Geometry check sheet. Reference: the model listing, model coordinates, mm. Face numbers are marked on the shaded views. A direction names the side the tool comes from. Coordinates: 2 decimals unless noted, no trailing zeros. Order: outer loops, then holes, each group sorted by start corner. A loop starts at its lowest first (then second) coordinate and runs counter-clockwise, first axis right, second up. Notation, with made-up numbers: (0.25, -4.5) -> (16.25, -4.5) arc R28 ccw to (16.25, 19.5) -> close; hole circle Ø9 at (-19, -3.75). An arc over 180 degrees is marked (long way). Answer in a Markdown table with one row per item. Add a question column.
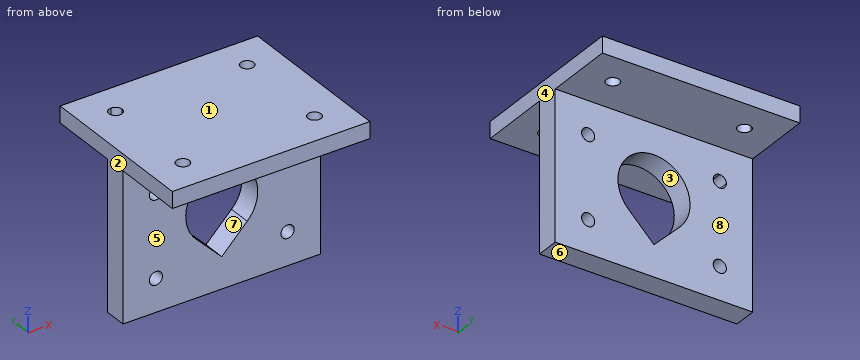
```python
from build123d import *

# Parameters (mm, degrees)
SKETCH_2_W           = 60
SKETCH_2_H           = 50
SKETCH_2_R           = 10.85
EXTRUDE_1_DEPTH      = 7
SKETCH_4_W           = 60
SKETCH_4_H           = 5
EXTRUDE_2_DEPTH      = 25
SKETCH_6_R           = 2
CUT_EXTRUDE_1_DEPTH  = 50
SKETCH_8_R           = 2
CUT_EXTRUDE_4_DEPTH  = 50
SKETCH_10_R          = 10.95
CUT_EXTRUDE_5_DEPTH  = 10
SKETCH_14_R          = 10.95
CUT_EXTRUDE_12_DEPTH = 10


with BuildPart() as part:
    # 草图2 → 凸台-拉伸1 (new body)
    with BuildSketch(Plane(origin=(0, 0, 0), x_dir=(1, 0, 0), z_dir=(0, 1, 0))):
        Rectangle(SKETCH_2_W, SKETCH_2_H)
        with Locations(Location((0, 0, 0), (0, 0, 270))):
            Circle(SKETCH_2_R, mode=Mode.SUBTRACT)
    extrude(amount=EXTRUDE_1_DEPTH)

    # 草图4 → 凸台-拉伸2 (add, symmetric)
    with BuildSketch(Plane(origin=(0, 3, 0), x_dir=(1, 0, 0), z_dir=(0, 1, 0))):
        with Locations((0, -22.5)):
            Rectangle(SKETCH_4_W, SKETCH_4_H)
    extrude(amount=EXTRUDE_2_DEPTH, both=True)

    # 草图6 → 切除-拉伸1 (cut)
    with BuildSketch(Plane.XY.offset(25)):
        with BuildLine():
            ThreePointArc((-18, 18), (-18.585786438, 19.414213562), (-20, 20))
            Line((-20, 20), (-20, 18))
            Line((-20, 18), (-22, 18))
            ThreePointArc((-22, 18), (-20, 16), (-18, 18))
        make_face()
        with BuildLine():
            Line((-20, 18), (-20, 20))
            ThreePointArc((-20, 20), (-21.414213562, 19.414213562), (-22, 18))
            Line((-22, 18), (-20, 18))
        make_face()
        with Locations((20, 18)):
            Circle(SKETCH_6_R)
        with Locations((-20, -12)):
            Circle(SKETCH_6_R)
        with Locations((20, -12)):
            Circle(SKETCH_6_R)
    extrude(amount=-CUT_EXTRUDE_1_DEPTH, mode=Mode.SUBTRACT)

    # 草图8 → 切除-拉伸4 (cut)
    with BuildSketch(Plane.XZ):
        with BuildLine():
            ThreePointArc((-18, 10), (-18.585786438, 11.414213562), (-20, 12))
            Line((-20, 12), (-20, 10))
            Line((-20, 10), (-22, 10))
            ThreePointArc((-22, 10), (-20, 8), (-18, 10))
        make_face()
        with BuildLine():
            Line((-20, 10), (-20, 12))
            ThreePointArc((-20, 12), (-21.414213562, 11.414213562), (-22, 10))
            Line((-22, 10), (-20, 10))
        make_face()
        with Locations(Location((20, 10, 0), (0, 0, 270))):
            Circle(SKETCH_8_R)
        with Locations(Location((20, -15, 0), (0, 0, 270))):
            Circle(SKETCH_8_R)
        with Locations(Location((-20, -15, 0), (0, 0, 270))):
            Circle(SKETCH_8_R)
    extrude(amount=-CUT_EXTRUDE_4_DEPTH, mode=Mode.SUBTRACT)

    # 草图10 → 切除-拉伸5 (cut)
    with BuildSketch(Plane(origin=(0, 7, 0), x_dir=(1, 0, 0), z_dir=(0, 1, 0))):
        with Locations(Location((0, 0, 0), (0, 0, 270))):
            Circle(SKETCH_10_R)
    extrude(amount=-CUT_EXTRUDE_5_DEPTH, mode=Mode.SUBTRACT)

    # 草图14 → 切除-拉伸12 (cut)
    with BuildSketch(Plane(origin=(0, 7, 0), x_dir=(1, 0, 0), z_dir=(0, 1, 0))):
        with BuildLine():
            ThreePointArc((-7.742819254, 7.742819254), (-4.190383584, 10.116480881), (0, 10.95))
            Line((0, 10.95), (0, 15.485638508))
            Line((0, 15.485638508), (-7.742819254, 7.742819254))
        make_face()
        with BuildLine():
            Line((0, 15.485638508), (0, 10.95))
            ThreePointArc((0, 10.95), (4.190383584, 10.116480881), (7.742819254, 7.742819254))
            Line((7.742819254, 7.742819254), (0, 15.485638508))
        make_face()
        Circle(SKETCH_14_R)
    extrude(amount=-CUT_EXTRUDE_12_DEPTH, mode=Mode.SUBTRACT)


solid = part.part
```
(1) Mould release check, pull along X, two halves, no side actions. Record for the marked faces 1, 2 and 3: +X half, -X half, draft (parallel to the pull), parting line (faces both ways), or undercut.
(2) Cross-section at A-A (z = 0). Enter the section's corners in (x, y), plus the area to 3 significant figures.
(3) Cross-section at B-B (x = 20). Enter the section's corners in (y, z).
(4) Scan lines: line 1 along Y through (x, z) = (20, 21); line 2 along Z through (x, y) = (0, 2); line 3 along Z through (x, y) = (-25, -10). Record each from-to range of solid material in increasing order.
(5) Cross-section at C-C (x = -7). Enter the section's corners in (y, z).
(6) Go/stop test with flat-tipped pins: P1, Ø17.5, axis at x = 13.5, y = -10.5, coming from the -Z side; P2, Ø4.5, axis at x = -20, z = -15, coming from the +Y side; P3, Ø6.5, axis at x = 20, y = -12, coming from the +Z side. Record where each tip stops, or that it passes through.
(7) Cross-section at D-D (z = 5.5). Enter the section's corners in (x, y), plus the area to 3 significant figures.
(8) Access from +Z, -Z, +X, -X, +Y, -Y to the whole of each face (thin tool, end or side, straight path). Record for the marked faces 4, 5, 6, 7 and 8.
Checks:
| question | item | result |
|---|---|---|
| 1 | face 1 | draft |
| 1 | face 2 | -X half |
| 1 | face 3 | undercut |
| 2 | outline | (-30, 0) -> (-10.95, 0) -> (-10.95, 7) -> (-30, 7) -> close; (10.95, 0) -> (30, 0) -> (30, 7) -> (10.95, 7) -> close |
| 2 | area | 267 mm² |
| 3 | outline | (-22, 20) -> (-14, 20) -> (-14, 25) -> (-22, 25) -> close; (-10, 20) -> (0, 20) -> (0, 12) -> (7, 12) -> (7, 20) -> (16, 20) -> (16, 25) -> (-10, 25) -> close; (0, -25) -> (7, -25) -> (7, -17) -> (0, -17) -> close; (0, -13) -> (7, -13) -> (7, 8) -> (0, 8) -> close; (20, 20) -> (28, 20) -> (28, 25) -> (20, 25) -> close |
| 4 | line 1 | -22 to -14, -10 to 16, 20 to 28 |
| 4 | line 2 | -25 to -15.49, 10.95 to 25 |
| 4 | line 3 | 20 to 25 |
| 5 | outline | (-22, 20) -> (0, 20) -> (0, 8.42) -> (7, 8.42) -> (7, 20) -> (28, 20) -> (28, 25) -> (-22, 25) -> close; (0, -25) -> (7, -25) -> (7, -8.49) -> (0, -8.49) -> close |
| 6 | P1 | z = 20 |
| 6 | P2 | y = 7 |
| 6 | P3 | z = 25 |
| 7 | outline | (-30, 0) -> (-9.47, 0) -> (-9.47, 7) -> (-30, 7) -> close; (9.47, 0) -> (30, 0) -> (30, 7) -> (9.47, 7) -> close |
| 7 | area | 287 mm² |
| 8 | face 4 | +Z, -Z, +X, +Y, -Y |
| 8 | face 5 | -Z, +X, -X, -Y |
| 8 | face 6 | -Z, +X, -X, +Y, -Y |
| 8 | face 7 | +Y, -Y |
| 8 | face 8 | -Z, +X, -X, +Y |
